Verification items for the finished model (mm, model axes). Coordinates: 2 decimals unless noted, no trailing zeros. Order: outer loops, then holes, each group sorted by start corner. A loop starts at its lowest first (then second) coordinate and runs counter-clockwise, first axis right, second up. Notation, with made-up numbers: M -16,82.25 L -3,82.25 A36 cw -3,119.25 Z; hole C -36.75,-30.75 d5. An arc over 180 degrees is marked long. Write item = value, one per line.
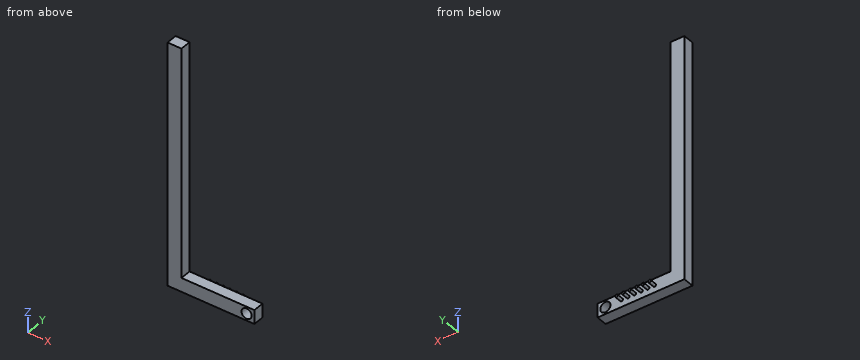
```python
from build123d import *

# Parameters (mm, degrees)
SKETCH1_R           = 1.47
BOSS_EXTRUDE1_DEPTH = 3.14
SKETCH6_R           = 0.4
BOSS_EXTRUDE4_DEPTH = 2


with BuildPart() as part:
    # Sketch1 → Boss-Extrude1 (new body)
    with BuildSketch(Plane(origin=(0, 0, 0), x_dir=(1, 0, 0), z_dir=(0, 1, 0))):
        Polygon((12.5, 2), (12.5, -2), (-8.5, -2), (-8.5, -68), (-12.5, -68), (-12.5, 2), (-8.5, 2), align=None)
        with Locations(Location((10.25, 0, 0), (0, 0, 270))):
            Circle(SKETCH1_R, mode=Mode.SUBTRACT)
    extrude(amount=BOSS_EXTRUDE1_DEPTH)

    # Sketch6 → Boss-Extrude4 (add)
    with BuildSketch(Plane(origin=(0, 3.14, 0), x_dir=(1, 0, 0), z_dir=(0, 1, 0))):
        with Locations(Location((-3.935899676, -0.003030319, 0), (0, 0, 90))):
            Circle(SKETCH6_R)
        with Locations(Location((-2.03089972, -0.002623383, 0), (0, 0, 90))):
            Circle(SKETCH6_R)
        with Locations(Location((-0.125899763, -0.002216446, 0), (0, 0, 90))):
            Circle(SKETCH6_R)
        with Locations(Location((1.779100193, -0.00180951, 0), (0, 0, 90))):
            Circle(SKETCH6_R)
        with Locations(Location((3.68410015, -0.001402574, 0), (0, 0, 90))):
            Circle(SKETCH6_R)
        with Locations(Location((5.589100106, -0.000995637, 0), (0, 0, 90))):
            Circle(SKETCH6_R)
    extrude(amount=BOSS_EXTRUDE4_DEPTH)


solid = part.part
```
Item 1: Sectioned sample at C-C, the plane y = 4.5. Enter the section's corners in (x, z).
Report:
outline = C -3.94,0 d0.8; C -2.03,0 d0.8; C -0.13,0 d0.8; C 1.78,0 d0.8; C 3.68,0 d0.8; C 5.59,0 d0.8
Item 2: Sectioned sample at D-D, the plane z = 61.5. Enter the section's corners in (x, y), then the cut area to 3 significant figures.
Report:
outline = M -12.5,0 L -8.5,0 L -8.5,3.14 L -12.5,3.14 Z
area = 12.6 mm^2
Item 3: Sectioned sample at A-A, the plane x = 10.25. Enter the section's corners in (y, z).
Report:
outline = M 0,-2 L 3.14,-2 L 3.14,-1.47 L 0,-1.47 Z; M 0,1.47 L 3.14,1.47 L 3.14,2 L 0,2 Z
Item 4: Gauge pin test, flat ends, axial feed: pin 1 (12 mm diameter, centred on x = -3.5, z = 44, fed in from -Y); pin 2 (1 mm diameter, centred on y = 1.5, z = 17.5, fed in from +X). Record the tip position at first contact, or that the pin passes through.
Report:
pin_1 = 0
pin_2 = -8.5
Item 5: Sectioned sample at B-B, the plane y = 1.35. Enter the section's corners in (x, z), then the cut area to 3 significant figures.
Report:
outline = M -12.5,-2 L 12.5,-2 L 12.5,2 L -8.5,2 L -8.5,68 L -12.5,68 Z; hole C 10.25,0 d2.94
area = 357 mm^2
Item 6: Scan lines: L1, parallel to X at y = 1.45, z = 0; L2, parallel to Z at x = -7.75, y = 2.7; L3, parallel to X at y = 0.95, z = 30.5. Record each from-to range of solid material in increasing order. Write a range as from..to.
Report:
L1 = -12.5..8.78, 11.72..12.5
L2 = -2..2
L3 = -12.5..-8.5
